from build123d import *

# Parameters (mm, degrees)
BOSS_EXTRUDE1_DEPTH                             = 3
F_10_0_10_DIAMETER_HOLE1_D                      = 10
F_10_0_10_DIAMETER_HOLE1_DEPTH                  = 10
F_10_0_10_DIAMETER_HOLE1_TIP                    = 3.004303095
CIRPATTERN1_COUNT                               = 4
CSK_FOR_M3_FLAT_HEAD_MACHINE_SCREW1_D           = 3.2
CSK_FOR_M3_FLAT_HEAD_MACHINE_SCREW1_CSINK_D     = 5.7
CSK_FOR_M3_FLAT_HEAD_MACHINE_SCREW1_CSINK_ANGLE = 90


with BuildPart() as part:
    # Sketch1 → Boss-Extrude1 (new body)
    with BuildSketch(Plane(origin=(0, 0, 0), x_dir=(1, 0, 0), z_dir=(0, 1, 0))):
        with BuildLine():
            ThreePointArc((-3.5, -17), (0, -20.5), (3.5, -17))
            Line((3.5, -17), (3.5, -10.5))
            ThreePointArc((3.5, -10.5), (5.550252532, -5.550252532), (10.5, -3.5))
            Line((10.5, -3.5), (17, -3.5))
            ThreePointArc((17, -3.5), (20.5, 0), (17, 3.5))
            Line((17, 3.5), (10.5, 3.5))
            ThreePointArc((10.5, 3.5), (5.550252532, 5.550252532), (3.5, 10.5))
            Line((3.5, 10.5), (3.5, 17))
            ThreePointArc((3.5, 17), (0, 20.5), (-3.5, 17))
            Line((-3.5, 17), (-3.5, 10.5))
            ThreePointArc((-3.5, 10.5), (-5.550252532, 5.550252532), (-10.5, 3.5))
            Line((-10.5, 3.5), (-17, 3.5))
            ThreePointArc((-17, 3.5), (-20.5, 0), (-17, -3.5))
            Line((-17, -3.5), (-10.5, -3.5))
            ThreePointArc((-10.5, -3.5), (-5.550252532, -5.550252532), (-3.5, -10.5))
            Line((-3.5, -10.5), (-3.5, -17))
        make_face()
    extrude(amount=BOSS_EXTRUDE1_DEPTH)

    # Ø10.0 (10) Diameter Hole1
    with Locations(Plane(origin=(0, 0, 0), x_dir=(0, 0, -1), z_dir=(0, -1, 0))):
        with Locations((0, 0)):
            Hole(F_10_0_10_DIAMETER_HOLE1_D / 2, depth=F_10_0_10_DIAMETER_HOLE1_DEPTH)
            with Locations((0, 0, -(F_10_0_10_DIAMETER_HOLE1_DEPTH + F_10_0_10_DIAMETER_HOLE1_TIP / 2))):  # 118° drill point
                Cone(0, F_10_0_10_DIAMETER_HOLE1_D / 2, F_10_0_10_DIAMETER_HOLE1_TIP, mode=Mode.SUBTRACT)

    # Sketch8 → Ø3.2 (3.2) Diameter Hole3 (revolve, cut)
    with BuildSketch(Plane(origin=(0, 0, 17), x_dir=(0, 0, -1), z_dir=(1, 0, 0))):
        Polygon((0, 0), (0, 10.96137699), (1.6, 10), (1.6, 0), align=None)
    f_3_2_3_2_diameter_hole3 = revolve(axis=Axis((0, -6.35, 17), (0, 1, 0)), mode=Mode.SUBTRACT)

    # CirPattern1: Ø3.2 (3.2) Diameter Hole3 ×4 about axis
    cirpattern1_axis = Axis((0, 0, 0), (0, 1, 0))
    for i in range(1, CIRPATTERN1_COUNT):
        add(f_3_2_3_2_diameter_hole3.rotate(cirpattern1_axis, i * 360 / CIRPATTERN1_COUNT), mode=Mode.SUBTRACT)

    # CSK for M3 Flat Head Machine Screw1 (through all)
    with Locations(Plane(origin=(0, 0, -8), x_dir=(0, 0, -1), z_dir=(0, -1, 0))):
        with Locations((0, 0), (-16, 0), (-8, -9.5), (-8, 9.5)):
            CounterSinkHole(CSK_FOR_M3_FLAT_HEAD_MACHINE_SCREW1_D / 2, CSK_FOR_M3_FLAT_HEAD_MACHINE_SCREW1_CSINK_D / 2, counter_sink_angle=CSK_FOR_M3_FLAT_HEAD_MACHINE_SCREW1_CSINK_ANGLE)


solid = part.part
Input: part model. Units: mm. Frame: model coordinates. A direction names the side the tool comes from. Round coordinates to 2 decimals unless told otherwise and drop trailing zeros. Write each loop counter-clockwise with the first axis right and the second up, starting at its lowest first coordinate (ties: lowest second). Pieces come first, ordered by that corner, then holes.
1) Contact query for flat-ended pins moving along their axis: P1, Ø1.5, axis at x = -11.5, y = 1.5, coming from the +Z side; P2, Ø4, axis at x = 0, z = -17, coming from the +Y side; P3, Ø0.9, axis at y = 1.5, z = -13, coming from the +X side; P4, Ø1.9, axis at x = 0, z = 8, coming from the -Y side. Output: stop coordinate, or through.
2) Cut plane A-A (x = 0). Return the cut outline in (y, z), then the cut area to 3 significant figures.
3) Reachability of faces 5 (the flat face through (-14, 1, -3.5)), 6 (the flat face through (3.5, 1, 14)), 7 (the flat face through (-3, 0, -5)) from +Z, -Z, +X, -X, +Y, -Y: full face, straight path, thin tool, end or side. Return the list, or none.
4) Cut plane B-B (z = 0). Return the cut outline in (x, y), then the cut area to 3 significant figures.
5) Cut plane C-C (y = 2.4). Count the separate pieces of the cut face and the enclosed holes in it, then the cut area to 3 significant figures.
6) Cut plane D-D (z = 8). Return the cut outline in (x, y).
7) Draft query along X for faces 1 (the cylindrical face through (-5.5, 1.5, -5.6)), 2 (the cylindrical face through (-18.6, 1.48, -0.07)), 3 (the cylindrical face through (0.07, 1.48, -18.6)), 4 (the cylindrical face through (5.5, 1.5, 5.6)). Return one class per face: pulls with the +X half, pulls with the -X half, needs draft (parallel to the pull), parting line crosses it, or undercut.
8) Ray query, L1, parallel to X at y = 1.9, z = -17; L2, parallel to Z at x = 16, y = 1.9. Return the intervals inside material, ascending.
Geometry says:
1. P1: stops at z = 3.5
1. P2: stops at y = 3
1. P3: stops at x = 3.5
1. P4: passes through
2. outline: (0, -20.5) - (3, -20.5) - (3, -18.6) - (0, -18.6) - close; (0, -15.4) - (3, -15.4) - (3, -9.6) - (1.25, -9.6) - (0, -10.85) - close; (0, -5.15) - (1.25, -6.4) - (3, -6.4) - (3, -5) - (0, -5) - close; (0, 5) - (3, 5) - (3, 6.4) - (1.25, 6.4) - (0, 5.15) - close; (0, 10.85) - (1.25, 9.6) - (3, 9.6) - (3, 15.4) - (0, 15.4) - close; (0, 18.6) - (3, 18.6) - (3, 20.5) - (0, 20.5) - close
2. area: 51.5 mm2
3. face 5: -Z, -X, +Y, -Y
3. face 6: +Z, +X, +Y, -Y
3. face 7: +Z, -Z, +X, -X, -Y
4. outline: (-20.5, 0) - (-18.6, 0) - (-18.6, 3) - (-20.5, 3) - close; (-15.4, 0) - (-12.35, 0) - (-11.1, 1.25) - (-11.1, 3) - (-15.4, 3) - close; (-7.9, 1.25) - (-6.65, 0) - (-5, 0) - (-5, 3) - (-7.9, 3) - close; (5, 0) - (6.65, 0) - (7.9, 1.25) - (7.9, 3) - (5, 3) - close; (11.1, 1.25) - (12.35, 0) - (15.4, 0) - (15.4, 3) - (11.1, 3) - close; (18.6, 0) - (20.5, 0) - (20.5, 3) - (18.6, 3) - close
4. area: 51.5 mm2
5. separate pieces: 1
5. enclosed holes: 9
5. area: 403 mm2
6. outline: (-3.96, 0) - (-2.85, 0) - (-1.6, 1.25) - (-1.6, 3) - (-3.96, 3) - close; (1.6, 1.25) - (2.85, 0) - (3.96, 0) - (3.96, 3) - (1.6, 3) - close
7. face 1: pulls with the -X half
7. face 2: undercut
7. face 3: undercut
7. face 4: pulls with the +X half
8. L1: x = -3.5 to -1.6, 1.6 to 3.5
8. L2: z = -3.5 to -1.25, 1.25 to 3.5
